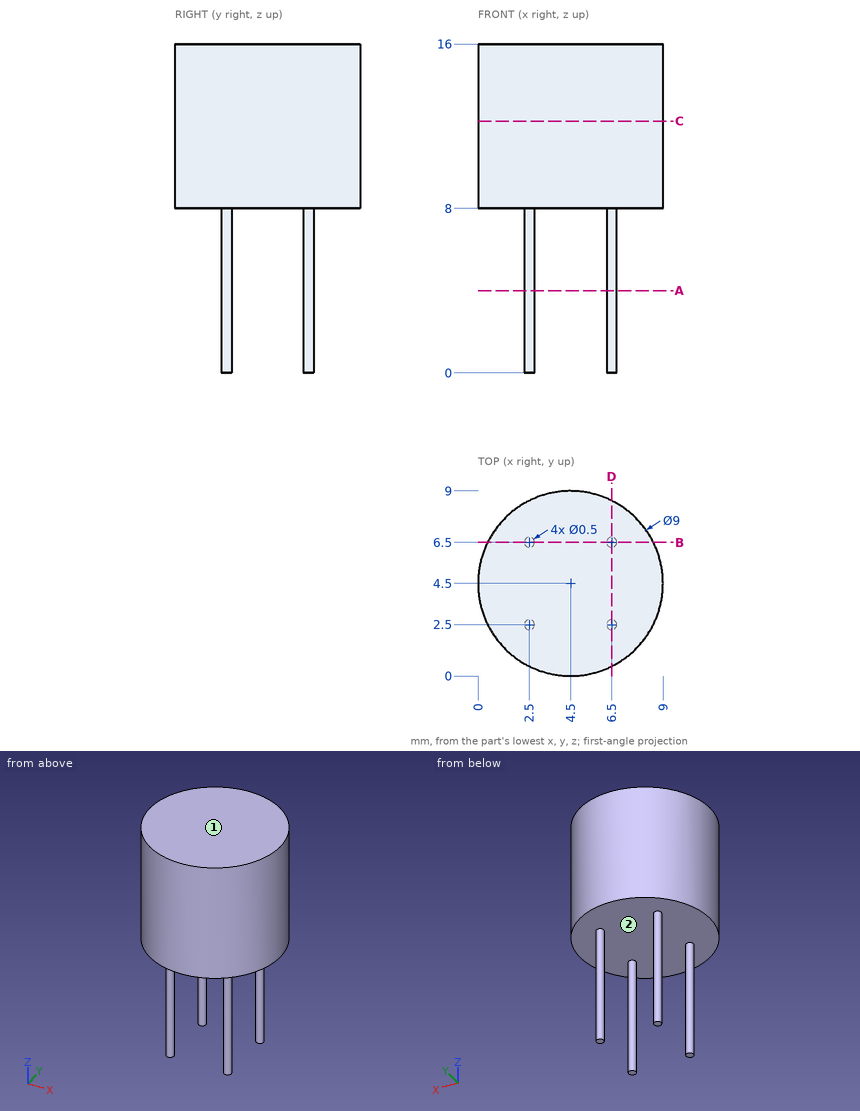
Verification items for this drawing (mm, ordinates from the low corner). A direction names the side the tool comes from. Give positions to 0.01 mm unless a question says otherwise; leave off trailing zeros. Write each loop counter-clockwise with the first axis right and the second up, starting at its lowest first coordinate (ties: lowest second). Pieces come first, ordered by that corner, then holes. Notation, with made-up numbers: (2, 40.5) - (16, 40.5) arc R27 cw to (16, 78.5) - close; hole circle Ø9 at (51.25, 77). An arc over 180 degrees is marked (long way). Answer as a JSON object with one key per item and string values. Group by question number.
1) Thickness scan on probe 1 along Z at (x, y) = (2.75, 3.5); probe 2 along Y at (x, z) = (1.5, 12.5); probe 3 along X at (y, z) = (6, 10.75). Record the ranges inside material, lowest first. Write a range as from..to.
2) Depth check by flat-ended pin: P1, Ø1, axis at y = 7, z = 12.5, coming from the -X side; P2, Ø1.5, axis at y = 6.5, z = 8.5, coming from the +X side; P3, Ø2, axis at x = 4.5, y = 6, coming from the -Z side. Enter the tip coordinate at first touch or a pass-through.
3) Sectioned sample at C-C (z = 12.25). Record the cut outline in (x, y), then the cut area to 3 significant figures.
4) Access from +Z, -Z, +X, -X, +Y, -Y to the whole of each face (thin tool, end or side, straight path). Record for the marked faces 1 and 2.
5) Sectioned sample at A-A (z = 4). Record the cut outline in (x, y), then the cut area to 3 significant figures.
6) Sectioned sample at B-B (y = 6.5). Record the cut outline in (x, z).
Geometry results:
{
 "1": {"probe 1": "z = 8..16", "probe 2": "y = 1.15..7.85", "probe 3": "x = 0.26..8.74"},
 "2": {"P1": "stops at x = 0.47", "P2": "stops at x = 8.82", "P3": "stops at z = 8"},
 "3": {"outline": "circle Ø9 at (4.5, 4.5)", "area": "63.6 mm^2"},
 "4": {"face 1": "+Z, +X, -X, +Y, -Y", "face 2": "-Z"},
 "5": {"outline": "circle Ø0.5 at (2.5, 2.5); circle Ø0.5 at (2.5, 6.5); circle Ø0.5 at (6.5, 2.5); circle Ø0.5 at (6.5, 6.5)", "area": "0.785 mm^2"},
 "6": {"outline": "(0.47, 8) - (2.25, 8) - (2.25, 0) - (2.75, 0) - (2.75, 8) - (6.25, 8) - (6.25, 0) - (6.75, 0) - (6.75, 8) - (8.53, 8) - (8.53, 16) - (0.47, 16) - close"}
}
